Input: part model. Units: mm. Frame: model coordinates. Face numbers are marked on the shaded views. Give positions to 0.01 mm unless a question says otherwise; leave off trailing zeros. Write each loop counter-clockwise with the first axis right and the second up, starting at its lowest first coordinate (ties: lowest second). Pieces come first, ordered by that corner, then holes.
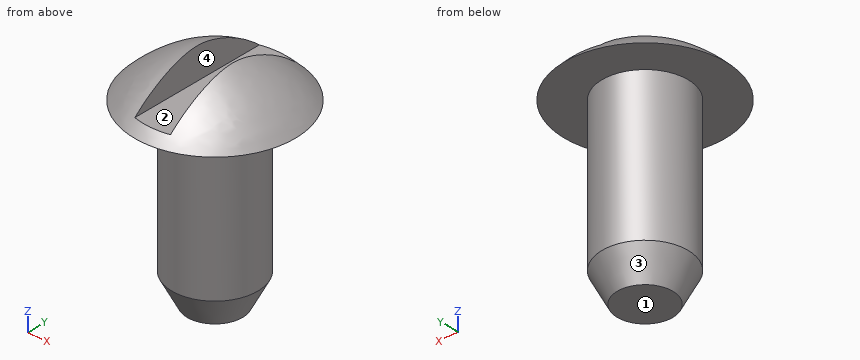
```python
from build123d import *

# Parameters (mm, degrees)
F3_W     = 2.54
F3_H     = 10.16
F4_DEPTH = 2.54


with BuildPart() as f1:
    # F0 (on Right) → F1 (revolve)
    with BuildSketch(Plane.YZ):
        with BuildLine():
            ThreePointArc((5.715, 12.7), (3.104294, 14.73173), (0, 15.875))
            Line((0, 15.875), (0, 0))
            Line((0, 0), (1.966236, 0))
            Line((1.966236, 0), (3.048, 2.089057))
            Line((3.048, 2.089057), (3.048, 12.7))
            Line((3.048, 12.7), (5.715, 12.7))
        make_face()
    revolve(axis=Axis((0, 0, 7.9375), (0, 0, -1)))

    # F3 (on offset) → F4 (cut)
    with BuildSketch(Plane.XY.offset(15.875)):
        Rectangle(F3_W, F3_H)
    extrude(amount=-F4_DEPTH, mode=Mode.SUBTRACT)


solid = f1.part
```
Item 1: Mould query, pull axis X, two halves, no side actions, for the marked faces 1, 2, 3 and 4. Classes: +X half, -X half, draft (parallel to the pull), parting line (faces both ways), or undercut.
Item 2: Section A-A (z = 9). Return loops of the section in (x, y).
Item 3: Pin query (flat end, axial travel): pin 1 (2.5 mm diameter, centred on y = 1.5, z = 15, fed in from +X); pin 2 (1.5 mm diameter, centred on x = 4.5, z = 14, fed in from +Y); pin 3 (3 mm diameter, centred on x = -3.5, y = 3, fed in from -Z). Return the tip coordinate at first contact, or that it passes through.
Item 4: Ray query, line 1 (Z direction, x = 0.75, y = -3.25) (3 decimals); line 2 (X direction, y = 2, z = 14); line 3 (X direction, y = 3.5, z = 12.75). Return the intervals inside material, ascending.
Solved:
1. face 1: draft
1. face 2: undercut
1. face 3: parting line
1. face 4: undercut
2. outline: circle Ø6.1 at (0, 0)
3. pin 1: stops at x = 4.37
3. pin 2: stops at y = 2.92
3. pin 3: stops at z = 12.7
4. line 1: z = 12.7 to 13.335
4. line 2: x = -3.75 to -1.27, 1.27 to 3.75
4. line 3: x = -4.46 to 4.46
